Input: dimensioned drawing with shaded views. Units: mm. Origin: part minimum x, y, z. Round coordinates to 2 decimals unless told otherwise and drop trailing zeros. Use one line per item in the form item = value. Start each with the question number.
Q1. Section A-A (x = 55). Give the number of separate pieces and of enclosed holes in the cut face.
Q2. Material intervals for probe 1 along X at (y, z) = (2.1, 20); probe 2 along X at (y, z) = (0.95, 18.75), sorted ascending.
Q3. Contact query for a flat-ended pin moving along its axis: pin 1 (4 mm diameter, centred on x = 55, z = 7.18, fed in from +Y). Output: stop coordinate, or through.
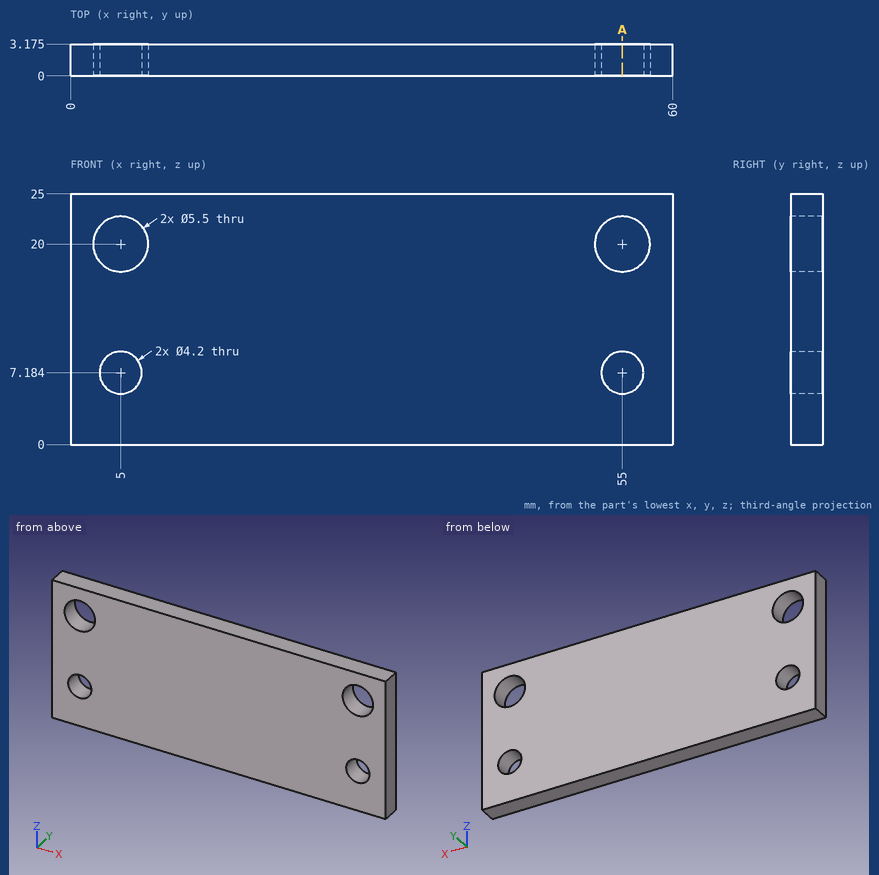
Results list:
q1.separate_pieces = 3
q1.enclosed_holes = 0
q2.probe_1 = 0 to 2.25, 7.75 to 52.25, 57.75 to 60
q2.probe_2 = 0 to 2.55, 7.45 to 52.55, 57.45 to 60
q3.pin_1 = through
